Solid Edge part; units mm, degrees
sketch "Sketch1" plane through (0, 0, 0) normal (0, -1, 0) x (1, 0, 0)
  line L0 (0, -32) -> (250, -32)
  line L1 (250, -32) -> (250, 0)
  line L2 (250, 0) -> (0, 0)
  line L3 (0, 0) -> (0, -32)
extrude "Protrusion1" add sketch "Sketch1" against normal blind 40
fillet "Round_1" [suppressed]
sketch "Sketch2" plane through (125, 0, -16) normal (0, -1, 0) x (1, 0, 0)
  line L0 (-60, 16) -> (-109.8999, 3.3905)
  arc A0 (-125, -16) -> (-109.8999, 3.3905) centre (-105, -16) cw
  line L1 (-125, 16) -> (-125, -16)
  line L2 (-60, 16) -> (-125, 16)
extrude "ExtrudedCutout_2" cut sketch "Sketch2" against normal blind 50
fillet "Round_2" radius 20 1 edges at (65, 20, 0)
Read the model definition and answer for the solid it produces. Units are mm, in the model's axes. Give positions to 0.01 mm unless a question says otherwise; leave off trailing zeros. Write each loop counter-clockwise with the first axis right and the second up, starting at its lowest first coordinate (ties: lowest second). Pieces come first, ordered by that corner, then holes. Notation, with made-up numbers: M 2,37.25 L 52,37.25 A29 cw 52,63.25 Z; hole C 68.5,-4 d5. An arc over 180 degrees is marked long. Put each result on its own line as item: value. Start each with the question number.
1. The part is cut by section A-A, the plane y = 13. Give the vertices of the cut face in (x, z).
2. Consider line 1 along X through (y, z) = (34.5, -26); line 2 along X through (y, z) = (3.5, -19.5); line 3 along Z through (x, y) = (57, 3). Determine where each line is inside the solid, lowest interval first.
3. The part is cut by section B-B, the plane x = 59. Give the vertices of the cut face in (y, z).
4. The part is cut by section C-C, the plane z = -17. Give the vertices of the cut face in (x, y).
Final values:
1. outline: M 0,-32 L 250,-32 L 250,0 L 67.49,0 A20 ccw 62.59,-0.61 L 15.1,-12.61 A20 ccw Z
2. line 1: x = 0.92 to 250
2. line 2: x = 4.39 to 250
2. line 3: z = -32 to -2.02
3. outline: M 0,-32 L 40,-32 L 40,-1.52 L 0,-1.52 Z
4. outline: M 6.77,0 L 250,0 L 250,40 L 6.77,40 Z
